```python
from build123d import *

# Parameters (mm, degrees)
SKETCH_1_W      = 25
SKETCH_1_H      = 3
EXTRUDE_1_DEPTH = 20
SKETCH_2_W      = 18
SKETCH_2_H      = 4
EXTRUDE_2_DEPTH = 3
EXTRUDE_3_DEPTH = 2
CHAMFER_1_SIZE  = 0.75
CHAMFER_2_SIZE  = 0.5
CHAMFER_3_SIZE  = 2
CHAMFER1_SIZE   = 2
FILLET1_R       = 1


with BuildPart() as part:
    # Эскиз1 → Бобышка-Вытянуть1 (new body)
    with BuildSketch(Plane.XY):
        with Locations((-4.579529598, 16.89)):
            Rectangle(SKETCH_1_W, SKETCH_1_H)
    extrude(amount=EXTRUDE_1_DEPTH)

    # Эскиз2 → Бобышка-Вытянуть2 (add)
    with BuildSketch(Plane(origin=(0, 18.39, 0), x_dir=(1, 0, 0), z_dir=(0, 1, 0))):
        with Locations((-4.579529598, -2)):
            Rectangle(SKETCH_2_W, SKETCH_2_H)
    extrude(amount=EXTRUDE_2_DEPTH)

    # Эскиз3 → Бобышка-Вытянуть3 (add)
    with BuildSketch(Plane(origin=(0, 0, 0), x_dir=(-1, 0, 0), z_dir=(0, 0, -1))):
        Polygon((-4.420470402, 21.39), (13.579529598, 21.39), (13.579529598, 19.89), (13.579529598, 18.896471803), (-4.420470402, 18.896471803), (-4.420470402, 19.89), align=None)
    extrude(amount=EXTRUDE_3_DEPTH)

    # Фаска1
    chamfer_1_edges = [part.edges().sort_by_distance(p)[0] for p in [
        (-4.579529598, 18.896471803, -2),
    ]]
    chamfer(chamfer_1_edges, length=CHAMFER_1_SIZE)

    # Фаска2
    chamfer_2_edges = [part.edges().sort_by_distance(p)[0] for p in [
        (-4.579529598, 21.39, -2),
    ]]
    chamfer(chamfer_2_edges, length=CHAMFER_2_SIZE)

    # Фаска3
    chamfer_3_edges = [part.edges().sort_by_distance(p)[0] for p in [
        (-4.579529598, 21.39, 4),
    ]]
    chamfer(chamfer_3_edges, length=CHAMFER_3_SIZE)

    # Зеркальное отражение1: part across plane


with BuildPart() as part_1:
    add(part.part)
    add(part.part.mirror(Plane.XY.offset(20)))

    # Chamfer1
    chamfer1_edges = [part_1.edges().sort_by_distance(p)[0] for p in [
        (4.420470402, 21.39, 39.75),
        (-13.579529598, 21.39, 39.75),
        (4.420470402, 21.39, 0.25),
        (-13.579529598, 21.39, 0.25),
    ]]
    chamfer(chamfer1_edges, length=CHAMFER1_SIZE)

    # Fillet1
    # the kernel refuses this fillet: 1 mm, written as the material it adds along each edge
    with BuildSketch(Plane(origin=(-13.579529598, 18.39, 6.5), x_dir=(-1, 0, 0), z_dir=(0, 0, -1))) as fillet1_piece_1_section:
        with BuildLine():
            CenterArc((FILLET1_R, FILLET1_R), FILLET1_R, 180, 90)
            Line((0, FILLET1_R), (0, 0))
            Line((0, 0), (FILLET1_R, 0))
        make_face()
    fillet1_piece_1 = extrude(amount=6.5, mode=Mode.PRIVATE)
    fillet1_piece_1 = split(fillet1_piece_1, bisect_by=Plane(origin=(-13.579529598, 17.64, 5.75), z_dir=(0, -0.7071067811865476, -0.7071067811865476)), keep=Keep.TOP, mode=Mode.PRIVATE)
    fillet1_piece_1 = fillet1_piece_1 - Plane(origin=(-13.579529598, 19.39, 5), x_dir=(0, 0, -1), z_dir=(1, 0, 0)) * Cylinder(1, 17, mode=Mode.PRIVATE)
    add(fillet1_piece_1)
    with BuildSketch(Plane(origin=(-13.579529598, 18.39, 6.5), x_dir=(-1, 0, 0), z_dir=(0, 0, -1))) as fillet1_piece_2_section:
        with BuildLine():
            CenterArc((FILLET1_R, FILLET1_R), FILLET1_R, 180, 90)
            Line((0, FILLET1_R), (0, 0))
            Line((0, 0), (FILLET1_R, 0))
        make_face()
    fillet1_piece_2 = extrude(amount=9, mode=Mode.PRIVATE)
    fillet1_piece_2 = split(fillet1_piece_2, bisect_by=Plane(origin=(-13.579529598, 14.768235901, 2.878235901), z_dir=(0, 0.7071067811865476, 0.7071067811865476)), keep=Keep.TOP, mode=Mode.PRIVATE)
    fillet1_piece_2 = split(fillet1_piece_2, bisect_by=Plane(origin=(-13.579529598, 18.896471803, 6.5), z_dir=(0, 1, 0)), keep=Keep.TOP, mode=Mode.PRIVATE)
    fillet1_piece_2 = split(fillet1_piece_2, bisect_by=Plane(origin=(-13.579529598, 18.39, 0), z_dir=(0, 0, -1)), keep=Keep.TOP, mode=Mode.PRIVATE)
    add(fillet1_piece_2)
    with BuildSketch(Plane(origin=(6.920470402, 18.39, 4), x_dir=(0, 1, 0), z_dir=(-1, 0, 0))) as fillet1_piece_3_section:
        with BuildLine():
            CenterArc((FILLET1_R, -FILLET1_R), FILLET1_R, 90, 90)
            Line((0, -FILLET1_R), (0, 0))
            Line((0, 0), (FILLET1_R, 0))
        make_face()
    fillet1_piece_3 = extrude(amount=23, mode=Mode.PRIVATE)
    fillet1_piece_3 = split(fillet1_piece_3, bisect_by=Plane(origin=(6.170470402, 17.64, 4), z_dir=(-0.7071067811865476, -0.7071067811865476, 0)), keep=Keep.TOP, mode=Mode.PRIVATE)
    fillet1_piece_3 = split(fillet1_piece_3, bisect_by=Plane(origin=(-3.829529598, 29.14, 4), z_dir=(0.7071067811865476, -0.7071067811865476, 0)), keep=Keep.TOP, mode=Mode.PRIVATE)
    fillet1_piece_3 = fillet1_piece_3 - Plane(origin=(-14.579529598, 19.39, 4), x_dir=(0, -1, 0), z_dir=(0, 0, 1)) * Cylinder(1, 50, mode=Mode.PRIVATE)
    fillet1_piece_3 = fillet1_piece_3 - Plane(origin=(5.420470402, 19.39, 4), x_dir=(-1, 0, 0), z_dir=(0, 0, -1)) * Cylinder(1, 50, mode=Mode.PRIVATE)
    add(fillet1_piece_3)
    with BuildSketch(Plane(origin=(4.420470402, 18.39, -2.5), x_dir=(0, 1, 0), z_dir=(0, 0, 1))) as fillet1_piece_4_section:
        with BuildLine():
            CenterArc((FILLET1_R, -FILLET1_R), FILLET1_R, 90, 90)
            Line((0, -FILLET1_R), (0, 0))
            Line((0, 0), (FILLET1_R, 0))
        make_face()
    fillet1_piece_4 = extrude(amount=9, mode=Mode.PRIVATE)
    fillet1_piece_4 = split(fillet1_piece_4, bisect_by=Plane(origin=(4.420470402, 19.268235901, -1.621764099), z_dir=(0, 0.7071067811865476, 0.7071067811865476)), keep=Keep.TOP, mode=Mode.PRIVATE)
    fillet1_piece_4 = split(fillet1_piece_4, bisect_by=Plane(origin=(4.420470402, 18.896471803, -2.5), z_dir=(0, 1, 0)), keep=Keep.TOP, mode=Mode.PRIVATE)
    fillet1_piece_4 = split(fillet1_piece_4, bisect_by=Plane(origin=(4.420470402, 22.14, 1.25), z_dir=(0, -0.7071067811865476, -0.7071067811865476)), keep=Keep.TOP, mode=Mode.PRIVATE)
    fillet1_piece_4 = fillet1_piece_4 - Plane(origin=(4.420470402, 19.39, 5), x_dir=(0, 0, -1), z_dir=(1, 0, 0)) * Cylinder(1, 22, mode=Mode.PRIVATE)
    add(fillet1_piece_4)
    with BuildSketch(Plane(origin=(4.420470402, 18.39, 0), x_dir=(0, 1, 0), z_dir=(0, 0, 1))) as fillet1_piece_5_section:
        with BuildLine():
            CenterArc((FILLET1_R, -FILLET1_R), FILLET1_R, 90, 90)
            Line((0, -FILLET1_R), (0, 0))
            Line((0, 0), (FILLET1_R, 0))
        make_face()
    fillet1_piece_5 = extrude(amount=6.5, mode=Mode.PRIVATE)
    fillet1_piece_5 = split(fillet1_piece_5, bisect_by=Plane(origin=(4.420470402, 20.89, 2.5), z_dir=(0, -0.7071067811865476, -0.7071067811865476)), keep=Keep.TOP, mode=Mode.PRIVATE)
    fillet1_piece_5 = fillet1_piece_5 - Plane(origin=(4.420470402, 19.39, 5), x_dir=(0, 0, -1), z_dir=(1, 0, 0)) * Cylinder(1, 17, mode=Mode.PRIVATE)
    add(fillet1_piece_5)
    with BuildSketch(Plane(origin=(-13.579529598, 18.39, 33.5), x_dir=(-1, 0, 0), z_dir=(0, 0, 1))) as fillet1_piece_6_section:
        with BuildLine():
            CenterArc((FILLET1_R, -FILLET1_R), FILLET1_R, 90, 90)
            Line((0, -FILLET1_R), (0, 0))
            Line((0, 0), (FILLET1_R, 0))
        make_face()
    fillet1_piece_6 = extrude(amount=6.5, mode=Mode.PRIVATE)
    fillet1_piece_6 = split(fillet1_piece_6, bisect_by=Plane(origin=(-13.579529598, 17.64, 34.25), z_dir=(0, -0.7071067811865476, 0.7071067811865476)), keep=Keep.TOP, mode=Mode.PRIVATE)
    fillet1_piece_6 = fillet1_piece_6 - Plane(origin=(-13.579529598, 19.39, 35), x_dir=(0, -1, 0), z_dir=(1, 0, 0)) * Cylinder(1, 17, mode=Mode.PRIVATE)
    add(fillet1_piece_6)
    with BuildSketch(Plane(origin=(-13.579529598, 18.39, 36), x_dir=(-1, 0, 0), z_dir=(0, 0, 1))) as fillet1_piece_7_section:
        with BuildLine():
            CenterArc((FILLET1_R, -FILLET1_R), FILLET1_R, 90, 90)
            Line((0, -FILLET1_R), (0, 0))
            Line((0, 0), (FILLET1_R, 0))
        make_face()
    fillet1_piece_7 = extrude(amount=6.5, mode=Mode.PRIVATE)
    fillet1_piece_7 = split(fillet1_piece_7, bisect_by=Plane(origin=(-13.579529598, 18.896471803, 36), z_dir=(0, 1, 0)), keep=Keep.TOP, mode=Mode.PRIVATE)
    fillet1_piece_7 = split(fillet1_piece_7, bisect_by=Plane(origin=(-13.579529598, 16.018235901, 38.371764099), z_dir=(0, 0.7071067811865476, -0.7071067811865476)), keep=Keep.TOP, mode=Mode.PRIVATE)
    add(fillet1_piece_7)
    with BuildSketch(Plane(origin=(6.920470402, 18.39, 36), x_dir=(0, 0, -1), z_dir=(-1, 0, 0))) as fillet1_piece_8_section:
        with BuildLine():
            CenterArc((FILLET1_R, -FILLET1_R), FILLET1_R, 90, 90)
            Line((0, -FILLET1_R), (0, 0))
            Line((0, 0), (FILLET1_R, 0))
        make_face()
    fillet1_piece_8 = extrude(amount=23, mode=Mode.PRIVATE)
    fillet1_piece_8 = split(fillet1_piece_8, bisect_by=Plane(origin=(-3.829529598, 29.14, 36), z_dir=(0.7071067811865476, -0.7071067811865476, 0)), keep=Keep.TOP, mode=Mode.PRIVATE)
    fillet1_piece_8 = split(fillet1_piece_8, bisect_by=Plane(origin=(6.170470402, 17.64, 36), z_dir=(-0.7071067811865476, -0.7071067811865476, 0)), keep=Keep.TOP, mode=Mode.PRIVATE)
    fillet1_piece_8 = fillet1_piece_8 - Plane(origin=(-14.579529598, 19.39, 36), x_dir=(0, -1, 0), z_dir=(0, 0, -1)) * Cylinder(1, 50, mode=Mode.PRIVATE)
    fillet1_piece_8 = fillet1_piece_8 - Plane(origin=(5.420470402, 19.39, 36), x_dir=(0, -1, 0), z_dir=(0, 0, 1)) * Cylinder(1, 50, mode=Mode.PRIVATE)
    add(fillet1_piece_8)
    with BuildSketch(Plane(origin=(4.420470402, 18.39, 42.5), x_dir=(1, 0, 0), z_dir=(0, 0, -1))) as fillet1_piece_9_section:
        with BuildLine():
            CenterArc((FILLET1_R, -FILLET1_R), FILLET1_R, 90, 90)
            Line((0, -FILLET1_R), (0, 0))
            Line((0, 0), (FILLET1_R, 0))
        make_face()
    fillet1_piece_9 = extrude(amount=9, mode=Mode.PRIVATE)
    fillet1_piece_9 = split(fillet1_piece_9, bisect_by=Plane(origin=(4.420470402, 18.896471803, 42.5), z_dir=(0, 1, 0)), keep=Keep.TOP, mode=Mode.PRIVATE)
    fillet1_piece_9 = split(fillet1_piece_9, bisect_by=Plane(origin=(4.420470402, 19.268235901, 41.621764099), z_dir=(0, 0.7071067811865476, -0.7071067811865476)), keep=Keep.TOP, mode=Mode.PRIVATE)
    fillet1_piece_9 = split(fillet1_piece_9, bisect_by=Plane(origin=(4.420470402, 22.14, 38.75), z_dir=(0, -0.7071067811865476, 0.7071067811865476)), keep=Keep.TOP, mode=Mode.PRIVATE)
    fillet1_piece_9 = fillet1_piece_9 - Plane(origin=(4.420470402, 19.39, 35), x_dir=(0, -1, 0), z_dir=(1, 0, 0)) * Cylinder(1, 22, mode=Mode.PRIVATE)
    add(fillet1_piece_9)
    with BuildSketch(Plane(origin=(4.420470402, 18.39, 40), x_dir=(1, 0, 0), z_dir=(0, 0, -1))) as fillet1_piece_10_section:
        with BuildLine():
            CenterArc((FILLET1_R, -FILLET1_R), FILLET1_R, 90, 90)
            Line((0, -FILLET1_R), (0, 0))
            Line((0, 0), (FILLET1_R, 0))
        make_face()
    fillet1_piece_10 = extrude(amount=6.5, mode=Mode.PRIVATE)
    fillet1_piece_10 = split(fillet1_piece_10, bisect_by=Plane(origin=(4.420470402, 20.89, 37.5), z_dir=(0, -0.7071067811865476, 0.7071067811865476)), keep=Keep.TOP, mode=Mode.PRIVATE)
    fillet1_piece_10 = fillet1_piece_10 - Plane(origin=(4.420470402, 19.39, 35), x_dir=(0, -1, 0), z_dir=(1, 0, 0)) * Cylinder(1, 17, mode=Mode.PRIVATE)
    add(fillet1_piece_10)


solid = part_1.part
```
Check sheet for the modelled part. Datum: model origin and axes. Units: mm. A direction names the side the tool comes from. Coordinates: 2 decimals unless noted, no trailing zeros. Write each loop counter-clockwise with the first axis right and the second up, starting at its lowest first coordinate (ties: lowest second). Pieces come first, ordered by that corner, then holes. Notation, with made-up numbers: M 66,31.5 L 114,31.5 A13 ccw 114,36.5 Z; hole C 19.5,22.25 d4. An arc over 180 degrees is marked long. Write item = value, one per line. Start each with the question number.
1. Thickness scan on probe 1 along Y at (x, z) = (-0.25, 24.5); probe 2 along Z at (x, y) = (-8, 16.5); probe 3 along Z at (x, y) = (-9, 19.25). Record the ranges inside material, lowest first.
2. Mould release check, pull along Z, two halves, no side actions. Record for faces 1 (the cylindrical face through (-13.865, 18.691, 1.675)), 2 (the flat face through (-5, 18.39, 20)), 3 (the flat face through (-5, 17, 0)): pulls with the +Z half, pulls with the -Z half, needs draft (parallel to the pull), parting line crosses it, or undercut.
3. Tool access check on faces 4 (the flat face through (-4, 18.896, -1)), 5 (the flat face through (-4, 21.39, 0)), 6 (the flat face through (-4.71, 20.38, 36.99)). Record the directions out of +Z, -Z, +X, -X, +Y, -Y that give a thin tool (end or side, any length) a straight path to the whole face; none if there is none.
4. Sectioned sample at D-D (y = 16). Record the cut outline in (x, z), then the cut area to 3 significant figures.
5. Sectioned sample at B-B (y = 20.25). Record the cut outline in (x, z), then the cut area to 3 significant figures.
6. Sectioned sample at A-A (x = -3.5). Record the cut outline in (y, z), then the cut area to 3 significant figures.
7. Sectioned sample at C-C (z = 14). Record the cut outline in (x, y).
8. Go/stop test with flat-tipped pins: pin 1 (0.6 mm diameter, centred on x = -8, z = -0.5, fed in from -Y); pin 2 (6 mm diameter, centred on x = -2, z = 22.5, fed in from +Y); pin 3 (1.1 mm diameter, centred on x = -4.5, y = 17, fed in from -Z). Record where each tip stops, or that it passes through.
The answers:
q1.probe_1 = 15.39 to 18.39
q1.probe_2 = 0 to 40
q1.probe_3 = -1.6 to 4.01, 35.99 to 41.6
q2.face_1 = needs draft
q2.face_2 = undercut
q2.face_3 = pulls with the -Z half
q3.face_4 = -Z, +X, -X, -Y
q3.face_5 = +Z, -Z, +X, -X, +Y
q3.face_6 = +X, -X, +Y
q4.outline = M -17.08,0 L 7.92,0 L 7.92,40 L -17.08,40 Z
q4.area = 1,000 mm²
q5.outline = M -12.72,-2 L 3.56,-2 L 3.56,3.14 L -12.72,3.14 Z; M -12.72,36.86 L 3.56,36.86 L 3.56,42 L -12.72,42 Z
q5.area = 167 mm²
q6.outline = M 15.39,0 L 18.9,0 L 18.9,-1.25 L 19.65,-2 L 20.89,-2 L 21.39,-1.5 L 21.39,2 L 19.39,4 A1 cw 18.39,5 L 18.39,35 A1 cw 19.39,36 L 21.39,38 L 21.39,41.5 L 20.89,42 L 19.65,42 L 18.9,41.25 L 18.9,40 L 15.39,40 Z
q6.area = 150 mm²
q7.outline = M -17.08,15.39 L 7.92,15.39 L 7.92,18.39 L -17.08,18.39 Z
q8.pin_1 = 18.9
q8.pin_2 = 18.39
q8.pin_3 = 0
